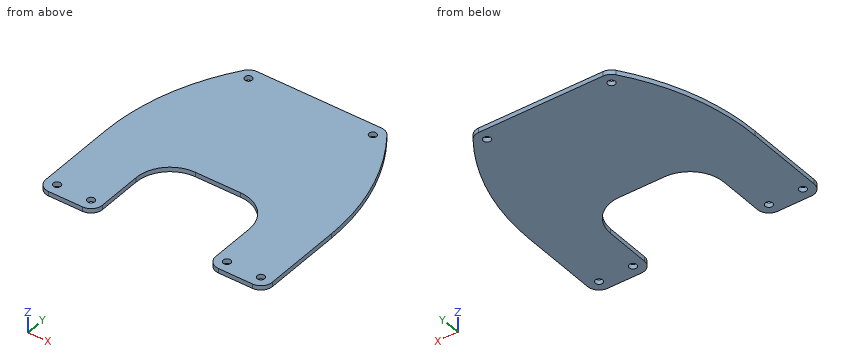
from build123d import *

# Parameters (mm, degrees)
SKETCH_1_W          = 25
SKETCH_1_H          = 40
EXTRUDE_1_DEPTH     = 2
FILLET_1_R          = 15
FILLET_2_R          = 5
FILLET_3_R          = 5
SKETCH_2_R          = 1.65
CUT_EXTRUDE_2_DEPTH = 2


with BuildPart() as part:
    # 草图1 → 凸台-拉伸1 (new body)
    with BuildSketch(Plane.XY):
        with BuildLine():
            Line((-25, 40), (0, 40))
            ThreePointArc((0, 40), (-5.131670195, 71.622776602), (-20, 100))
            Line((-20, 100), (-80, 100))
            ThreePointArc((-80, 100), (-94.868329805, 71.622776602), (-100, 40))
            Line((-100, 40), (-75, 40))
            Line((-75, 40), (-25, 40))
        make_face()
        with Locations((-87.5, 20)):
            Rectangle(SKETCH_1_W, SKETCH_1_H)
        with Locations((-12.5, 20)):
            Rectangle(SKETCH_1_W, SKETCH_1_H)
    extrude(amount=EXTRUDE_1_DEPTH)

    # 圆角1
    fillet_1_edges = [part.edges().sort_by_distance(p)[0] for p in [
        (-75, 40, 1),
        (-25, 40, 1),
    ]]
    fillet(fillet_1_edges, radius=FILLET_1_R)

    # 圆角2
    fillet_2_edges = [part.edges().sort_by_distance(p)[0] for p in [
        (-75, 0, 1),
        (-100, 0, 1),
        (0, 0, 1),
        (-25, 0, 1),
    ]]
    fillet(fillet_2_edges, radius=FILLET_2_R)

    # 圆角3
    fillet_3_edges = [part.edges().sort_by_distance(p)[0] for p in [
        (-80, 100, 1),
        (-20, 100, 1),
    ]]
    fillet(fillet_3_edges, radius=FILLET_3_R)

    # 草图2 → 切除-拉伸2 (cut)
    with BuildSketch(Plane.XY.offset(2)):
        with Locations((-77.459666924, 95)):
            Circle(SKETCH_2_R)
        with Locations((-22.540333076, 95)):
            Circle(SKETCH_2_R)
        with Locations((-95, 5)):
            Circle(SKETCH_2_R)
        with Locations((-5, 5)):
            Circle(SKETCH_2_R)
        with Locations((-80, 5)):
            Circle(SKETCH_2_R)
        with Locations((-20, 5)):
            Circle(SKETCH_2_R)
    extrude(amount=-CUT_EXTRUDE_2_DEPTH, mode=Mode.SUBTRACT)


solid = part.part
The listing builds one solid part. Answer for the finished solid, in the listing's coordinates (mm). Coordinates: 2 decimals unless noted, no trailing zeros. Loops run counter-clockwise (first coordinate to the right, second up) from the corner with the lowest first, then second, coordinate; pieces in that order, holes last. Notation, with made-up numbers: M 79.25,49.5 L 123.25,49.5 A28 cw 123.25,67.5 Z; hole C 65,16 d5. An arc over 180 degrees is marked long. Answer in a Markdown table with one row per item.
1) Find section B-B (y = 18). Determine the outline of the cut face in (x, z).
Answers below:
| item | result |
|---|---|
| outline | M -100,0 L -75,0 L -75,2 L -100,2 Z; M -25,0 L 0,0 L 0,2 L -25,2 Z |
2) Find section A-A (z = 1.05). Determine the outline of the cut face in (x, y), then the cut area to 3 significant figures.
Answers below:
| item | result |
|---|---|
| outline | M -100,5 A5 ccw -95,0 L -80,0 A5 ccw -75,5 L -75,25 A15 cw -60,40 L -40,40 A15 cw -25,25 L -25,5 A5 ccw -20,0 L -5,0 A5 ccw 0,5 L 0,40 A100 ccw -18.46,97.89 A5 ccw -22.54,100 L -77.46,100 A5 ccw -81.54,97.89 A100 ccw -100,40 Z; hole C -95,5 d3.3; hole C -80,5 d3.3; hole C -77.46,95 d3.3; hole C -22.54,95 d3.3; hole C -20,5 d3.3; hole C -5,5 d3.3 |
| area | 7,260 mm^2 |
3) Find section D-D (x = -42.5). Determine the outline of the cut face in (y, z).
Answers below:
| item | result |
|---|---|
| outline | M 40,0 L 100,0 L 100,2 L 40,2 Z |
4) Find the intervals of material crossed by probe 1 along Y at (x, z) = (-59.5, 0.1); probe 2 along X at (y, z) = (34.5, 0.8); probe 3 along X at (y, z) = (31, 1.8), in increasing order.
Answers below:
| item | result |
|---|---|
| probe 1 | 40 to 100 |
| probe 2 | -100 to -71.61, -28.39 to 0 |
| probe 3 | -100 to -73.75, -26.25 to 0 |
5) Find section C-C (y = 95). Determine the outline of the cut face in (x, z).
Answers below:
| item | result |
|---|---|
| outline | M -83.52,0 L -79.11,0 L -79.11,2 L -83.52,2 Z; M -75.81,0 L -24.19,0 L -24.19,2 L -75.81,2 Z; M -20.89,0 L -16.48,0 L -16.48,2 L -20.89,2 Z |
